Autodesk Inventor part; units mm, degrees
ref_plane "YZ Plane" through (0, 0, 0) normal (1, 0, 0) x (0, 1, 0)
ref_plane "XZ Plane" through (0, 0, 0) normal (0, 1, 0) x (-1, 0, 0)
ref_plane "XY Plane" through (0, 0, 0) normal (0, 0, 1) x (1, 0, 0)
sketch "Sketch1" plane through (0, 0, 0) normal (0, 1, 0) x (-1, 0, 0)
  line L0 (0, 0) -> (2, 0)
  line L1 (2, 0) -> (2, 90)
  line L2 (2, 90) -> (0, 90)
  line L3 (0, 90) -> (0, 0)
  line L4 (0, 0) -> (3.5, 0)
  line L5 (3.5, 0) -> (3.5, -4)
  line L6 (3.5, -4) -> (0, -4)
  line L7 (0, -4) -> (0, 0)
  dimension "d0" = 2
  dimension "d1" = 90
  dimension "d2" = 3.5
  dimension "d3" = 4
revolve "Revolution1" add sketch "Sketch1" angle 360 about axis through (0, 0, 90) along (0, 0, -1)
chamfer "Chamfer1" distance 0.5 angle 45 2 edges at (2, 0, 90) (3.5, 0, -4)
thread "Thread1"
sketch "Sketch2" plane through (0, 0, -4) normal (0, 0, -1) x (-1, 0, 0)
  line L0 (0, 0) -> (1.5, 0)
  line L1 (0, 0) -> (0.75, 1.299)
  line L2 (0, 0) -> (-0.75, 1.299)
  line L3 (0, 0) -> (-1.5, 0)
  line L4 (0, 0) -> (-0.75, -1.299)
  line L5 (0, 0) -> (0.75, -1.299)
  line L6 (0.75, 1.299) -> (1.5, 0)
  line L7 (1.5, 0) -> (0.75, -1.299)
  circle A0 centre (0, 0) radius 1.5
  line L8 (0.75, -1.299) -> (-0.75, -1.299)
  line L9 (-0.75, -1.299) -> (-1.5, 0)
  line L10 (-1.5, 0) -> (-0.75, 1.299)
  line L11 (-0.75, 1.299) -> (0.75, 1.299)
  dimension "d10" = 1.5
  dimension "d13" = 360
extrude "Extrusion1" cut sketch "Sketch2" against normal blind 2 contours L1 L6 L0 | L2 L11 L1 | L3 L10 L2 | L4 L9 L3 | L5 L8 L4 | L0 L7 L5
properties part number "screw_4_90"
Read the model definition and answer for the solid it produces. Units are mm, in the model's axes. A direction names the side the tool comes from. Coordinates: 2 decimals unless noted, no trailing zeros. Write each loop counter-clockwise with the first axis right and the second up, starting at its lowest first coordinate (ties: lowest second). Pieces come first, ordered by that corner, then holes. Notation, with made-up numbers: (9.25, 49.5) -> (54.25, 49.5) arc R17 ccw to (54.25, 60.5) -> close; hole circle Ø1 at (57, 45). An arc over 180 degrees is marked (long way). Write item = value, one per line.
(1) For a pull along X with two mould halves and no side action, classify faces 1 (the face through (0, 1.299, -3)), 2 (the face through (-3.233, -1.341, -1.774)), 3 (the face through (-1.3, 0.7, -4)) as +X half, -X half, draft (parallel to the pull), parting line (faces both ways), or undercut.
From the geometry:
face_1 = undercut
face_2 = parting line
face_3 = draft
(2) Which of the six approach directions +Z, -Z, +X, -X, +Y, -Y give full straight-line access (tool end or side, diameter ignored) to faces 4 (the face through (-2, -2, 0)), 5 (the face through (0, 0, 90)), 6 (the face through (0, 0, -2))?
From the geometry:
face_4 = +Z
face_5 = +Z, +X, -X, +Y, -Y
face_6 = -Z
(3) Straight lines are drawn through the part: L1, parallel to Z at x = 2.5, y = 1; L2, parallel to Z at x = -1, y = 0.75; L3, parallel to X at y = 0.25, z = 71. For each, find the intervals that lie inside material, in ascending order. Write a range as from..to.
From the geometry:
L1 = -4..0
L2 = -2..90
L3 = -1.98..1.98
(4) Section A-A on z = 46 is taken. Write down the section's boundary in (x, y).
From the geometry:
outline = circle Ø4 at (0, 0)
(5) Given pin 1 Ø2 at (x, z) = (2.5, 6.5) entering from -Y; pin 2 Ø3 at (x, z) = (-2.5, 67.5) entering from -Y; pin 3 Ø3 at (y, z) = (1.5, 31) entering from -X, each flat-ended and moving along its own axis, determine where each tip first touches the part or whether it passes through.
From the geometry:
pin_1 = -1.32
pin_2 = -1.73
pin_3 = -2
